Could you check a few things on this drawing? It's one solid part, dimensions in mm from its lowest x, y, z. Coordinates: 2 decimals unless noted, no trailing zeros. One line per question, with ' | ' between items.
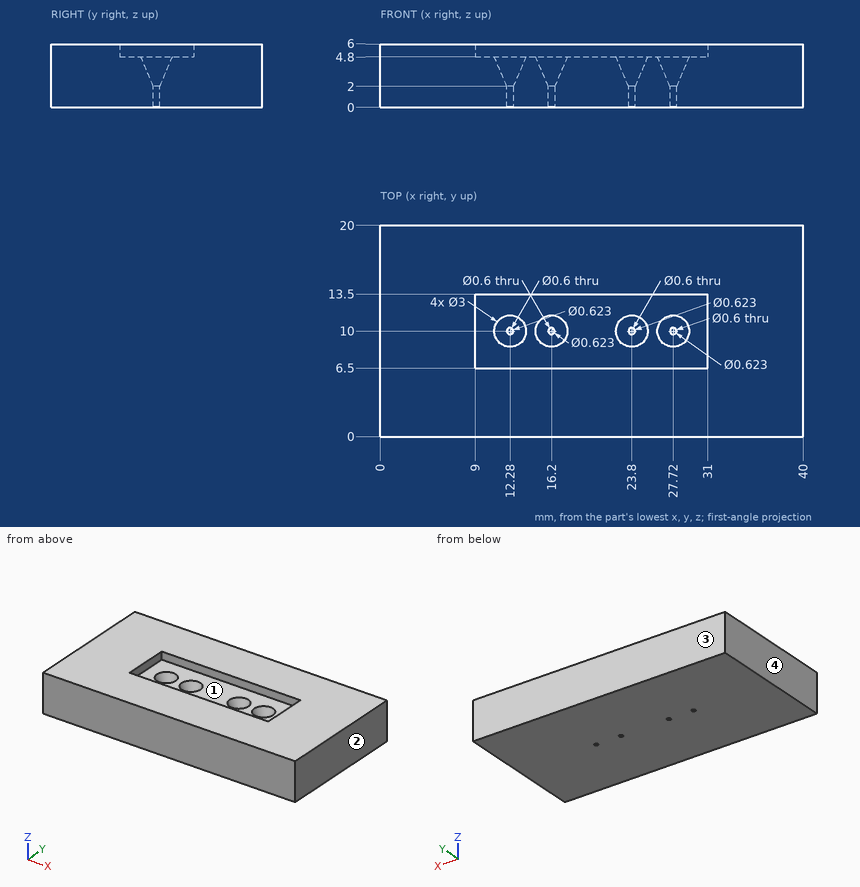
1) I'm going to push flat-ended pins straight in: pin 1 Ø0.5 at (x, y) = (24, 10) entering from +Z; pin 2 Ø3 at (x, y) = (28, 2.5) entering from -Z; pin 3 Ø3.5 at (x, y) = (19.5, 9) entering from +Z; pin 4 Ø0.7 at (x, y) = (27.5, 10) entering from +Z. Where does each tip first touch, or does it pass through?
Data:
pin 1: z = 2.33 | pin 2: z = 0 | pin 3: z = 4.8 | pin 4: z = 2.61
2) I need wall thicknesses on line 1 along X through (y, z) = (10.75, 4.6); line 2 along X through (y, z) = (7.5, 5.1); line 3 along X through (y, z) = (10.5, 4.1). Which ranges of each line are inside material? Lowest first, please. Write a range as from..to.
Data:
line 1: 0..11.08, 13.48..15, 17.4..22.6, 25..26.52, 28.92..40 | line 2: 0..9, 31..40 | line 3: 0..11.19, 13.37..15.11, 17.29..22.71, 24.89..26.63, 28.81..40
3) We'd pull the mould along X, two halves only. Please class the marked faces 1, 2, 3 and 4: pulls with the +X half, pulls with the -X half, needs draft (parallel to the pull), parting line crosses it, or undercut.
Data:
face 1: undercut | face 2: pulls with the +X half | face 3: needs draft | face 4: pulls with the -X half
